Part print with two shaded views. Sizes in mm from the minimum x, y, z corner. Give positions to 0.01 mm unless a question says otherwise; leave off trailing zeros. Order: outer loops, then holes, each group sorted by start corner. A loop starts at its lowest first (then second) coordinate and runs counter-clockwise, first axis right, second up.
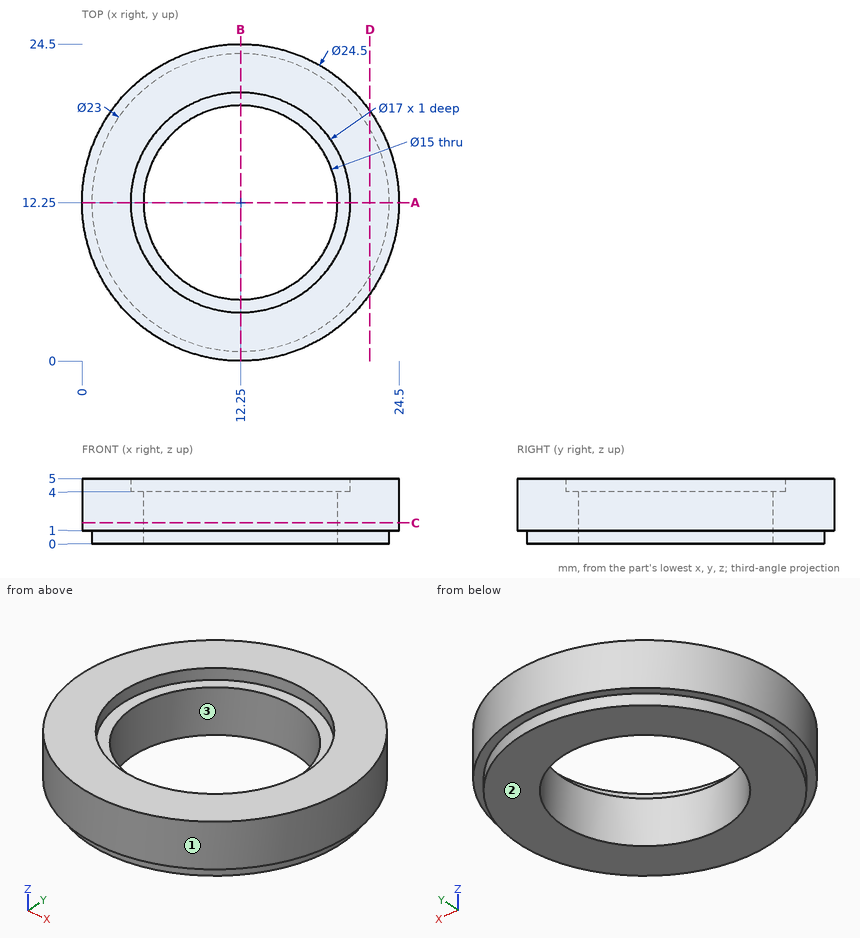
1. Wall check: line 1 (Y direction, x = 12.25, z = 4.3); line 2 (Y direction, x = 12.25, z = 2.1); line 3 (X direction, y = 13, z = 3.95). Give the ranges that are in metal, low to high.
2. Pin check, flat tip, straight feed: P1, Ø2, axis at y = 20.5, z = 3.5, coming from the +X side. Stop position of the tip, or through.
3. Mould opens along Y. For the marked faces 1, 2 and 3 say: released by +Y, released by -Y, zero draft, split by the parting line, or undercut.
4. Saw through at C-C on z = 1.6. Give the cut face in (x, y).
5. Saw through at D-D on x = 22.25. Give the cut face in (y, z), plus the area to 3 significant figures.
6. Saw through at A-A on y = 12.25. Give the cut face in (x, z), plus the area to 3 significant figures.
Reported:
1. line 1: y = 0 to 3.75, 20.75 to 24.5
1. line 2: y = 0 to 4.75, 19.75 to 24.5
1. line 3: x = 0.02 to 4.79, 19.71 to 24.48
2. P1: stops at x = 22.12
3. face 1: split by the parting line
3. face 2: zero draft
3. face 3: undercut
4. outline: circle Ø24.5 at (12.25, 12.25); hole circle Ø15 at (12.25, 12.25)
5. outline: (5.17, 1) - (6.57, 1) - (6.57, 0) - (17.93, 0) - (17.93, 1) - (19.33, 1) - (19.33, 5) - (5.17, 5) - close
5. area: 68.0 mm2
6. outline: (0, 1) - (0.75, 1) - (0.75, 0) - (4.75, 0) - (4.75, 4) - (3.75, 4) - (3.75, 5) - (0, 5) - close; (19.75, 0) - (23.75, 0) - (23.75, 1) - (24.5, 1) - (24.5, 5) - (20.75, 5) - (20.75, 4) - (19.75, 4) - close
6. area: 44.0 mm2
